Autodesk Inventor part; units mm, degrees
ref_plane "YZ Plane" through (0, 0, 0) normal (1, 0, 0) x (0, 1, 0)
ref_plane "XZ Plane" through (0, 0, 0) normal (0, 1, 0) x (-1, 0, 0)
ref_plane "XY Plane" through (0, 0, 0) normal (0, 0, 1) x (1, 0, 0)
sketch "Sketch3" plane through (0, 0, 0) normal (0, 1, 0) x (-1, 0, 0)
  line L0 (0, 0) -> (28, 0)
  line L1 (28, 0) -> (28, -96)
  line L2 (28, -96) -> (0, -96)
  line L3 (0, -96) -> (0, 0)
  dimension "d6" = 28
  dimension "d7" = 96
extrude "Extrusion3" add sketch "Sketch3" along normal blind 4.5
sketch "Sketch4" plane through (0, 4.5, 0) normal (0, 1, 0) x (1, 0, 0)
  line L0 (0, 96) -> (-28, 96)
  line L1 (-28, 96) -> (-28, 0)
  line L2 (-28, 0) -> (0, 0)
  line L3 (0, 0) -> (0, 96)
  line L4 (-28, 0) -> (-20, 0)
  line L5 (-20, 0) -> (-20, 96)
  line L6 (-20, 96) -> (-28, 96)
  line L7 (-28, 96) -> (-28, 0)
  line L8 (0, 0) -> (-20, 0)
  line L9 (-20, 0) -> (-20, 6)
  line L10 (-20, 6) -> (0, 6)
  line L11 (0, 6) -> (0, 0)
  line L12 (0, 96) -> (-20, 96)
  line L13 (-20, 96) -> (-20, 90)
  line L14 (-20, 90) -> (0, 90)
  line L15 (0, 90) -> (0, 96)
  dimension "d10" = 8
  dimension "d11" = 6
  dimension "d12" = 6
extrude "Extrusion4" add sketch "Sketch4" along normal blind 54 contours L5 L2 L1 L0 | L3 L10 L5 L14
sketch "Sketch5" plane through (0, 4.5, 0) normal (0, 1, 0) x (1, 0, 0)
  line L0 (0, 6) -> (-20, 6)
  line L1 (-20, 6) -> (-20, 0)
  line L2 (-20, 0) -> (0, 0)
  line L3 (0, 0) -> (0, 6)
  circle A0 centre (-10, 0) radius 2
  line L4 (-20, 96) -> (-20, 90)
  line L5 (-20, 90) -> (0, 90)
  line L6 (0, 90) -> (0, 96)
  line L7 (0, 96) -> (-20, 96)
  circle A1 centre (-10, 96) radius 2
  point P0 (-8, 0)
  point P1 (-12, 0)
  dimension "d15" = 4
  dimension "d16" = 4
extrude "Extrusion5" cut sketch "Sketch5" against normal through all contours L2 A0 | A1 L7 | L7 A1 picked at (-9.3527, 0.1595)
sketch "Sketch6" plane through (0, 58.5, 0) normal (0, 1, 0) x (1, 0, 0)
  line L0 (-20, 6) -> (0, 6)
  line L1 (0, 6) -> (0, 90)
  line L2 (0, 90) -> (-20, 90)
  line L3 (-20, 90) -> (-20, 96)
  line L4 (-20, 96) -> (-28, 96)
  line L5 (-28, 96) -> (-28, 0)
  line L6 (-28, 0) -> (-20, 0)
  line L7 (-20, 0) -> (-20, 6)
  line L8 (0, 20) -> (-14, 20)
  line L9 (-14, 20) -> (-14, 76)
  line L10 (-14, 76) -> (0, 76)
  line L11 (0, 76) -> (0, 20)
  point P0 (0, 0)
  point P1 (0, 76)
  dimension "d19" = 14
  dimension "d21" = 14
  dimension "d22" = 14
extrude "Extrusion6" add sketch "Sketch6" along normal blind 15 contours L8 L9 L10 L1
properties part number "driver"
Design review of the part built by this model. Coordinates are the model's own, in mm. A direction names the side the tool comes from. Coordinates: 2 decimals unless noted, no trailing zeros. Loops run counter-clockwise (first coordinate to the right, second up) from the corner with the lowest first, then second, coordinate; pieces in that order, holes last. Notation, with made-up numbers: (15, 3.25) - (44, 3.25) arc R27 cw to (44, 23.25) - close; hole circle Ø7 at (-10.75, 34). An arc over 180 degrees is marked (long way). Use CSV: the item, a comma, the result in double quotes. Start each with the question number.
1. For faces 1 (the flat face through (-7, 66, -20)), 2 (the flat face through (-20, 31, -3)), 3 (the flat face through (-7, 66, -76)), 4 (the flat face through (-10, 31, -90)), list the 3-axis set-ups (+Z, -Z, +X, -X, +Y, -Y) from which the entire face can be reached by the end or side of a thin tool; tool diameter is ignored.
2. Add section D-D on x = -21.5. Give the boundary of the cut face in (y, z), plus the area to 3 significant figures.
3. Clearance check with flat-ended pins moving along their axes: pin 1 (15.5 mm diameter, centred on x = -8.5, y = 66.5, fed in from +Z); pin 2 (15.5 mm diameter, centred on x = -6.5, y = 66, fed in from -Z); pin 3 (3 mm diameter, centred on x = -6.5, z = -92.5, fed in from +Y). State where each tip first meets the part, or that it passes through.
4. Mouldability with a two-part tool opening along X and no side actions: class faces 5 (the cylindrical face through (-10, 2, -2)), 6 (the flat face through (-23, 29, 0)), 7 (the flat face through (-20, 31, -93)) as released by +X, released by -X, zero draft, split by the parting line, or undercut.
5. Add section A-A on x = -10. Give the boundary of the cut face in (y, z).
6. Add section C-C on z = -10. Give the boundary of the cut face in (x, y), plus the area to 3 significant figures.
7. To check wall thickness, follow probe 1 along Z at (x, y) = (-5.25, 50.5); probe 2 along X at (y, z) = (60, -58); probe 3 along Y at (x, z) = (-17, -74.5). State the ranges of each line that lie inside material, in increasing order.
8. Add section B-B on y = 44.5. Give the boundary of the cut face in (x, z), plus the area to 3 significant figures.
Resolved:
1,face 1,"+Z, +X, -X, +Y"
1,face 2,"+Z, +X, +Y"
1,face 3,"-Z, +X, -X, +Y"
1,face 4,"-Z, +X, +Y"
2,outline,"(0, -96) - (58.5, -96) - (58.5, 0) - (0, 0) - close"
2,area,"5,620 mm2"
3,pin 1,"z = -20"
3,pin 2,"z = -90"
3,pin 3,"y = 4.5"
4,face 5,"undercut"
4,face 6,"zero draft"
4,face 7,"released by +X"
5,outline,"(0, -94) - (4.5, -94) - (4.5, -90) - (58.5, -90) - (58.5, -76) - (73.5, -76) - (73.5, -20) - (58.5, -20) - (58.5, -6) - (4.5, -6) - (4.5, -2) - (0, -2) - close"
6,outline,"(-28, 0) - (0, 0) - (0, 58.5) - (-28, 58.5) - close"
6,area,"1,640 mm2"
7,probe 1,"-90 to -6"
7,probe 2,"-14 to 0"
7,probe 3,"0 to 58.5"
8,outline,"(-28, -96) - (-20, -96) - (-20, -90) - (0, -90) - (0, -6) - (-20, -6) - (-20, 0) - (-28, 0) - close"
8,area,"2,450 mm2"
